from build123d import *

# Parameters (mm, degrees)
F0_W     = 52
F0_H     = 32
F1_DEPTH = 9
F2_W     = 32
F2_H     = 6
F3_DEPTH = 32.001
F4_W     = 6
F4_H     = 32
F5_DEPTH = 50.5
F7_DEPTH = 12.001


with BuildPart() as f1:
    # F0 (on Front) → F1 (new body, symmetric)
    with BuildSketch(Plane.XZ):
        with Locations((-26, 16)):
            Rectangle(F0_W, F0_H)
    extrude(amount=F1_DEPTH, both=True)

    # F2 (on face) → F3 (cut, through all)
    with BuildSketch(Plane.XY.offset(32)):
        with Locations((-21, 0)):
            Rectangle(F2_W, F2_H)
    extrude(amount=-F3_DEPTH, mode=Mode.SUBTRACT)

    # F4 (on face) → F5 (join)
    with BuildSketch(Plane(origin=(-52, 0, 0), x_dir=(0, -1, 0), z_dir=(-1, 0, 0))):
        with Locations((0, 16)):
            Rectangle(F4_W, F4_H)
    extrude(amount=F5_DEPTH)

    # F6 (on face) → F7 (cut, through all)
    with BuildSketch(Plane.XZ.offset(3)):
        Polygon((-102.5, 28.5), (-99, 32), (-102.5, 32), align=None)
        Polygon((-102.5, 0), (-99, 0), (-102.5, 3.5), align=None)
    extrude(amount=-F7_DEPTH, mode=Mode.SUBTRACT)


solid = f1.part
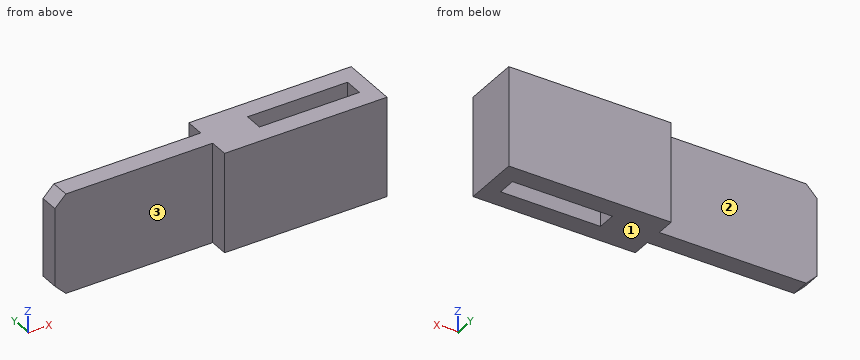
Here's how the part is built. I have some questions about the finished solid (model axes, mm). Face numbers are marked on the shaded views. A direction names the side the tool comes from. Round coordinates to 2 decimals unless told otherwise and drop trailing zeros. Order: outer loops, then holes, each group sorted by start corner. A loop starts at its lowest first (then second) coordinate and runs counter-clockwise, first axis right, second up. Notation, with made-up numbers: M 88,16.5 L 141,16.5 A9 ccw 141,22.5 Z; hole C -7.5,-32.75 d5. An arc over 180 degrees is marked long. Return JSON: item names as keys, results as strings. Group by question number.
1. Please list where these lines run through material, in increasing order: probe 1 along Y at (x, z) = (-10, 10); probe 2 along X at (y, z) = (-1, 3.5); probe 3 along X at (y, z) = (-6.25, 14.5).
2. If we section it at C-C on y = 1: List the corners of the cut face in (x, z) for me.
3. On a 3-axis mill with a long thin cutter (end or side, diameter ignored), from which of +Z, -Z, +X, -X, +Y, -Y can I reach the whole of each face in a straight line? I mean the marked faces 1, 2 and 3. Say none if no direction works.
4. If we section it at D-D on x = -79: List the corners of the cut face in (y, z) for me.
5. If we section it at B-B on x = -36: List the corners of the cut face in (y, z) for me, then the cut area to 3 significant figures.
6. If we section it at A-A on z = 25: List the corners of the cut face in (x, y) for me.
7. I'm going to push flat-ended pins straight in: pin 1 Ø1.8 at (y, z) = (-1, 15) entering from +X; pin 2 Ø6.5 at (y, z) = (7, 21) entering from -X; pin 3 Ø9.5 at (x, z) = (-77.5, 21.5) entering from -Y; pin 4 Ø16 at (x, z) = (-71, 17) entering from +Y. Where does each tip first touch, or does it pass through?
Reply:
{
 "1": {"probe 1": "-9 to -3, 3 to 9", "probe 2": "-102.5 to -37, -5 to 0", "probe 3": "-52 to 0"},
 "2": {"outline": "M -102.5,3.5 L -99,0 L -37,0 L -37,32 L -99,32 L -102.5,28.5 Z; M -5,0 L 0,0 L 0,32 L -5,32 Z"},
 "3": {"face 1": "-Z, +X, -X, +Y, -Y", "face 2": "+Z, -Z, -X, +Y", "face 3": "+Z, -Z, -X, -Y"},
 "4": {"outline": "M -3,0 L 3,0 L 3,32 L -3,32 Z"},
 "5": {"outline": "M -9,0 L -3,0 L -3,32 L -9,32 Z; M 3,0 L 9,0 L 9,32 L 3,32 Z", "area": "384 mm^2"},
 "6": {"outline": "M -102.5,-3 L -52,-3 L -52,-9 L 0,-9 L 0,9 L -52,9 L -52,3 L -102.5,3 Z; hole M -37,-3 L -5,-3 L -5,3 L -37,3 Z"},
 "7": {"pin 1": "x = 0", "pin 2": "x = -52", "pin 3": "y = -3", "pin 4": "y = 3"}
}
